Can you work these out from the model? Positions are in its coordinate system, mm. Face numbers are marked on the shaded views. A direction names the side the tool comes from. Give positions to 0.01 mm unless a question says otherwise; leave off trailing zeros. Write each loop counter-clockwise with the first axis right and the second up, starting at its lowest first coordinate (ties: lowest second). Pieces come first, ordered by that corner, then holes. Notation, with made-up numbers: M 37.5,68 L 66.5,68 A27 cw 66.5,90 Z; hole C 31.25,-40 d9. An arc over 180 degrees is marked long. Answer as CSV lines item,"result". Start each with the question number.
```python
from build123d import *

# Parameters (mm, degrees)
F0_R            = 38
F1_DEPTH        = 3
F2_R            = 38
F2_R_2          = 35
F3_DEPTH        = 27
F4_W            = 12
F4_H            = 23
F4_R            = 2.5
F5_DEPTH        = 3
F6_R            = 2
F8_DEPTH        = 15
F8_COPIES_COUNT = 8


# Not quite as in the source:
# - a pattern or mirror of a feature is missing from the dataset's text; its kind, count and spacing are read off the source's solid


with BuildPart() as f1:
    # F0 (on Top) → F1 (new body)
    with BuildSketch(Plane.XY):
        Circle(F0_R)
    extrude(amount=F1_DEPTH)

    # F2 (on face) → F3 (join)
    with BuildSketch(Plane.XY.offset(3)):
        Circle(F2_R)
        Circle(F2_R_2, mode=Mode.SUBTRACT)
    extrude(amount=F3_DEPTH)

    # F4 (on Top) → F5 (join)
    with BuildSketch(Plane.XY):
        with Locations((0, -41.5)):
            Rectangle(F4_W, F4_H)
        with Locations((0, -48)):
            Circle(F4_R, mode=Mode.SUBTRACT)
    extrude(amount=F5_DEPTH)

    # F6
    f6_edges = [f1.edges().sort_by_distance(p)[0] for p in [
        (6, -53, 1.5),
        (-6, -53, 1.5),
    ]]
    fillet(f6_edges, radius=F6_R)

    # F7 (on face) → F8 (cut)
    with BuildSketch(Plane.XY.offset(30)):
        with BuildLine():
            Line((-9.5144401541, 36.7896103344), (-8.7633001419, 33.8851674132))
            ThreePointArc((-8.7633001419, 33.8851674132), (0, 35), (8.7633001419, 33.8851674132))
            Line((8.7633001419, 33.8851674132), (9.5144401541, 36.7896103344))
            ThreePointArc((9.5144401541, 36.7896103344), (0, 38), (-9.5144401541, 36.7896103344))
        make_face()
    f8 = extrude(amount=-F8_DEPTH, mode=Mode.SUBTRACT)

    # F8_copies: F8 ×8 about axis
    f8_copies_axis = Axis((0, 0, 0), (0, 0, 1))
    for i in range(1, F8_COPIES_COUNT):
        add(f8.rotate(f8_copies_axis, i * 360 / F8_COPIES_COUNT), mode=Mode.SUBTRACT)


solid = f1.part
```
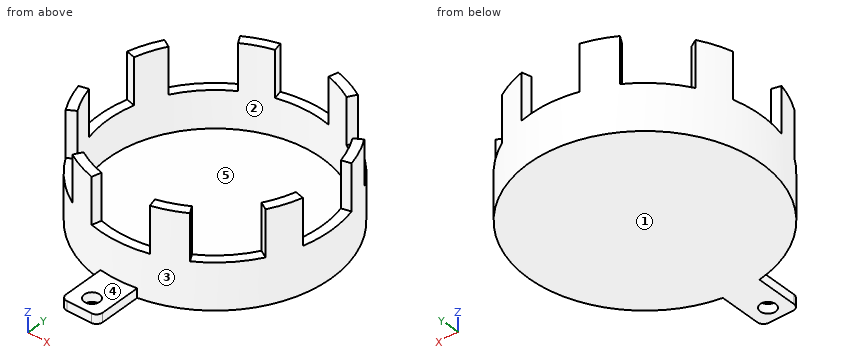
1) I want a section at D-D, the plane y = -48. Please give me the cut outline in (x, z).
2) I want a section at C-C, the plane y = 0. Please give me the cut outline in (x, z), then the cut area to 3 significant figures.
3) I want a section at B-B, the plane z = 28. State how many separate pieces and enclosed holes the cut face has, then the cut area to 3 significant figures.
4) On a 3-axis mill with a long thin cutter (end or side, diameter ignored), from which of +Z, -Z, +X, -X, +Y, -Y can I reach the whole of each face in a straight line? I mean the marked faces 1 and 2. Say none if no direction works.
5) I want a section at A-A, the plane x = 0. Please give me the cut outline in (y, z), then the cut area to 3 significant figures.
6) Thinking about a two-plate mould opening in Y: for the marked faces 3, 4 and 5, which applies, released by +Y, released by -Y, zero draft, split by the parting line, or undercut?
7) I'm going to push flat-ended pins straight in: P1, Ø0.9, axis at y = -43, z = 2, coming from the -X side; P2, Ø4.5, axis at x = -25.5, y = -22.5, coming from the +Z side; P3, Ø5, axis at x = 21, y = 23, coming from the -Z side; P4, Ø3, axis at x = 0, y = -48, coming from the -Z side. Where does each tip first touch, or does it pass through?
8) I need wall thicknesses on L1, parallel to X at y = 0, z = 14.5; L2, parallel to Z at x = -11.5, y = 2; L3, parallel to Y at x = 0, z = 2.35. Which ranges of each line are inside material? Lowest first, please. Write a range as from..to.
Values found:
1,outline,"M -6,0 L -2.5,0 L -2.5,3 L -6,3 Z; M 2.5,0 L 6,0 L 6,3 L 2.5,3 Z"
2,outline,"M -38,0 L 38,0 L 38,15 L 35,15 L 35,3 L -35,3 L -35,15 L -38,15 Z"
2,area,"300 mm²"
3,separate pieces,"8"
3,enclosed holes,"0"
3,area,"245 mm²"
4,face 1,"-Z, +X, -X, +Y, -Y"
4,face 2,"+Z"
5,outline,"M -53,0 L -50.5,0 L -50.5,3 L -53,3 Z; M -45.5,0 L 38,0 L 38,15 L 35,15 L 35,3 L -35,3 L -35,15 L -38,15 L -38,3 L -45.5,3 Z"
5,area,"330 mm²"
6,face 3,"split by the parting line"
6,face 4,"zero draft"
6,face 5,"undercut"
7,P1,"stops at x = -6"
7,P2,"stops at z = 15"
7,P3,"stops at z = 0"
7,P4,"passes through"
8,L1,"x = -38..-35, 35..38"
8,L2,"z = 0..3"
8,L3,"y = -53..-50.5, -45.5..38"
